Geometry: final body of the model. Coordinates: model frame, mm. Face numbers are marked on the shaded views. A direction names the side the tool comes from. Give positions to 0.01 mm unless a question says otherwise; leave off trailing zeros. Write each loop counter-clockwise with the first axis right and the second up, starting at its lowest first coordinate (ties: lowest second). Pieces come first, ordered by that corner, then holes.
Q1. Section C-C (y = 71.5). State how many separate pieces and enclosed holes the cut face has, plus the area to 3 significant figures.
Q2. Section A-A (x = 53). Return the cut outline in (y, z), plus the area to 4 significant figures.
Q3. Section B-B (z = 192). Return the cut outline in (x, y), plus the area to 3 significant figures.
Q4. Mould query, pull axis X, two halves, no side actions, for the marked faces 3, 4, 5 and 6. Classes: +X half, -X half, draft (parallel to the pull), parting line (faces both ways), or undercut.
Q5. Pin query (flat end, axial travel): pin 1 Ø13.5 at (x, z) = (139, 72) entering from -Y. Return the tip coordinate at first contact, or that it passes through.
Q6. Line query: line 1 (X direction, y = 85.5, z = 252); line 2 (Z direction, x = 18, y = 113); line 3 (Y direction, x = 156.5, z = 127.5). Output: solid intervals per line, ascending.
Q7. Reachability of the marked faces 1 and 2 from +Z, -Z, +X, -X, +Y, -Y: full face, straight path, thin tool, end or side. Return the list, or none.
from build123d import *

# Parameters (mm, degrees)
F0_W     = 300
F0_H     = 135
F1_DEPTH = 410
F2_W     = 105
F2_H     = 96.25
F2_W_2   = 70
F2_H_2   = 45.625
F3_DEPTH = 125


with BuildPart() as f1:
    # F0 (on Top) → F1 (new body)
    with BuildSketch(Plane.XY):
        with Locations((150, 67.5)):
            Rectangle(F0_W, F0_H)
    extrude(amount=F1_DEPTH)

    # F2 (on face) → F3 (cut)
    with BuildSketch(Plane.XZ):
        with Locations((242.5, 356.875)):
            Rectangle(F2_W, F2_H)
        with Locations((150, 230.3125)):
            Rectangle(F2_W_2, F2_H_2)
        with Locations((150, 280.9375)):
            Rectangle(F2_W_2, F2_H_2)
        with Locations((150, 331.5625)):
            Rectangle(F2_W_2, F2_H_2)
        with Locations((150, 382.1875)):
            Rectangle(F2_W_2, F2_H_2)
        with Locations((150, 179.6875)):
            Rectangle(F2_W_2, F2_H_2)
        with Locations((150, 129.0625)):
            Rectangle(F2_W_2, F2_H_2)
        with Locations((150, 78.4375)):
            Rectangle(F2_W_2, F2_H_2)
        with Locations((242.5, 53.125)):
            Rectangle(F2_W, F2_H)
        with Locations((150, 27.8125)):
            Rectangle(F2_W_2, F2_H_2)
        with Locations((57.5, 53.125)):
            Rectangle(F2_W, F2_H)
        with Locations((57.5, 154.375)):
            Rectangle(F2_W, F2_H)
        with Locations((57.5, 255.625)):
            Rectangle(F2_W, F2_H)
        with Locations((57.5, 356.875)):
            Rectangle(F2_W, F2_H)
        with Locations((242.5, 255.625)):
            Rectangle(F2_W, F2_H)
        with Locations((242.5, 154.375)):
            Rectangle(F2_W, F2_H)
    extrude(amount=-F3_DEPTH, mode=Mode.SUBTRACT)


solid = f1.part
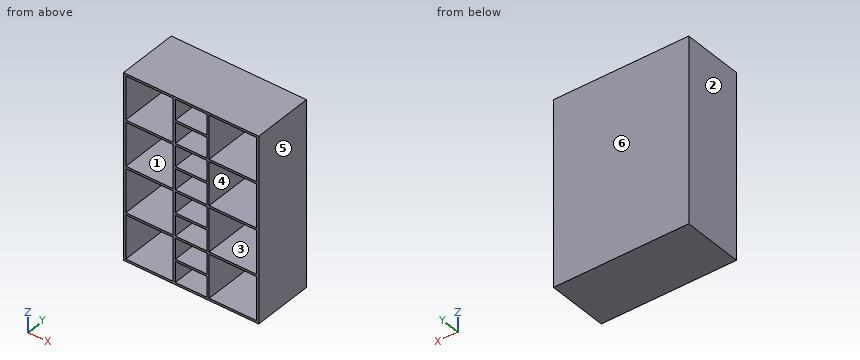
Computed:
1. separate pieces: 1
1. enclosed holes: 16
1. area: 16,600 mm2
2. outline: (0, 0) - (135, 0) - (135, 410) - (0, 410) - (0, 405) - (125, 405) - (125, 308.75) - (0, 308.75) - (0, 303.75) - (125, 303.75) - (125, 207.5) - (0, 207.5) - (0, 202.5) - (125, 202.5) - (125, 106.25) - (0, 106.25) - (0, 101.25) - (125, 101.25) - (125, 5) - (0, 5) - close
2. area: 7,225 mm2
3. outline: (0, 0) - (5, 0) - (5, 125) - (110, 125) - (110, 0) - (115, 0) - (115, 125) - (185, 125) - (185, 0) - (190, 0) - (190, 125) - (295, 125) - (295, 0) - (300, 0) - (300, 135) - (0, 135) - close
3. area: 5,500 mm2
4. face 3: undercut
4. face 4: undercut
4. face 5: +X half
4. face 6: draft
5. pin 1: stops at y = 125
6. line 1: x = 0 to 5, 110 to 115, 185 to 190, 295 to 300
6. line 2: z = 0 to 5, 101.25 to 106.25, 202.5 to 207.5, 303.75 to 308.75, 405 to 410
6. line 3: y = 125 to 135
7. face 1: -Y
7. face 2: +Z, -Z, -X, +Y, -Y
